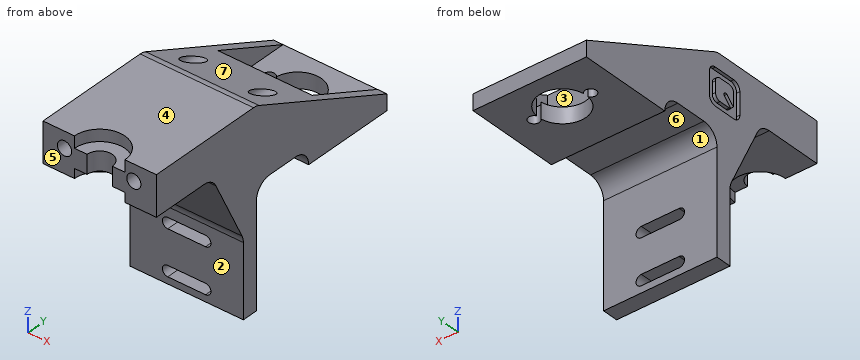
```python
from build123d import *

# Parameters (mm, degrees)
F0_W      = 30
F0_H      = 22
F1_DEPTH  = 5
F2_DEPTH  = 39.1
F3_W      = 30
F3_H      = 12.7
F4_DEPTH  = 50
F8_W      = 30
F8_H      = 5
F9_DEPTH  = 25
F10_W     = 30
F10_H     = 5
F11_DEPTH = 5
F12_W     = 30
F12_H     = 5
F13_DEPTH = 25
F15_DEPTH = 25
F16_DEPTH = 3
F18_DEPTH = 3
F19_DEPTH = 3
F21_DEPTH = 3
F23_DEPTH = 30
F24_R     = 2.25
F25_DEPTH = 500
F26_W     = 68.0921077728
F26_H     = 72.8289508261
F27_DEPTH = 25
F29_DEPTH = 36
F30_R     = 4.99999
F32_DEPTH = 1


# Not quite as in the source:
# - a fillet or chamfer is up to 0.001 mm smaller than in the source, because OpenCascade refuses the exact size


with BuildPart() as f1:
    # F0 (on Front) → F1 (new body)
    with BuildSketch(Plane.XZ):
        with Locations((0, 7.15)):
            Rectangle(F0_W, F0_H)
        with BuildLine():
            ThreePointArc((-6, -1.7), (-7.7, 0), (-6, 1.7))
            Line((-6, 1.7), (6, 1.7))
            ThreePointArc((6, 1.7), (7.7, 0), (6, -1.7))
            Line((6, -1.7), (-6, -1.7))
        make_face(mode=Mode.SUBTRACT)
        with BuildLine():
            ThreePointArc((-6, 12.6), (-7.7, 14.3), (-6, 16))
            Line((-6, 16), (6, 16))
            ThreePointArc((6, 16), (7.7, 14.3), (6, 12.6))
            Line((6, 12.6), (-6, 12.6))
        make_face(mode=Mode.SUBTRACT)
    extrude(amount=F1_DEPTH)

    # F2 (add): a face of the model
    f2_faces = [f1.faces().sort_by_distance(p)[0] for p in [
        (0, -2.5, 18.15),
    ]]
    extrude(f2_faces, amount=F2_DEPTH)

    # F3 (on face) → F4 (join)
    with BuildSketch(Plane.XZ.offset(5)):
        with Locations((0, 50.9)):
            Rectangle(F3_W, F3_H)
    extrude(amount=F4_DEPTH)

    # F6 (on offset) → F7 (revolve, cut)
    with BuildSketch(Plane.XZ.offset(38.3)):
        Polygon((8, 57.25), (0, 57.25), (0, 44.55), (8, 44.55), (8, 47.55), (4, 47.55), (4, 53.55), (8, 53.55), align=None)
    revolve(axis=Axis((0, -38.3, 50.9), (0, 0, 1)), mode=Mode.SUBTRACT)

    # F8 (on face) → F9 (join)
    with BuildSketch(Plane(origin=(0, 0, 0), x_dir=(-1, 0, 0), z_dir=(0, 1, 0))):
        with Locations((0, 36.45)):
            Rectangle(F8_W, F8_H)
    extrude(amount=F9_DEPTH)

    # F10 (on face) → F11 (join)
    with BuildSketch(Plane(origin=(0, 0, 33.95), x_dir=(1, 0, 0), z_dir=(0, 0, -1))):
        with Locations((0, -22.5)):
            Rectangle(F10_W, F10_H)
    extrude(amount=F11_DEPTH)

    # F12 (on face) → F13 (join)
    with BuildSketch(Plane(origin=(0, 25, 0), x_dir=(-1, 0, 0), z_dir=(0, 1, 0))):
        with Locations((0, 31.45)):
            Rectangle(F12_W, F12_H)
    extrude(amount=F13_DEPTH)

    # F14 (on face) → F15 (cut)
    with BuildSketch(Plane.XY.offset(33.95)):
        with BuildLine():
            ThreePointArc((7.4548611111, 38.3216117173), (0, 45), (-7.4548611111, 38.3216117173))
            ThreePointArc((-7.4548611111, 38.3216117173), (-10.75, 37.5), (-7.4548611111, 36.6783882827))
            ThreePointArc((-7.4548611111, 36.6783882827), (0, 30), (7.4548611111, 36.6783882827))
            ThreePointArc((7.4548611111, 36.6783882827), (10.75, 37.5), (7.4548611111, 38.3216117173))
        make_face()
    extrude(amount=-F15_DEPTH, mode=Mode.SUBTRACT)

    # F16 (add): a face of the model
    f16_faces = [f1.faces().sort_by_distance(p)[0] for p in [
        (15, -2.5, -2.6351662665),
    ]]
    extrude(f16_faces, amount=F16_DEPTH)

    # F17 (on face) → F18 (join)
    with BuildSketch(Plane.YZ.offset(18)):
        Polygon((50, 33.95), (0, 57.25), (0, 38.95), (25, 38.95), (25, 33.95), align=None)
    extrude(amount=-F18_DEPTH)

    # F19 (add): a face of the model
    f19_faces = [f1.faces().sort_by_distance(p)[0] for p in [
        (-15, -2.5, -2.6351662665),
    ]]
    extrude(f19_faces, amount=F19_DEPTH)

    # F20 (on face) → F21 (join)
    with BuildSketch(Plane(origin=(-18, 0, 0), x_dir=(0, -1, 0), z_dir=(-1, 0, 0))):
        Polygon((0, 57.25), (-50, 33.95), (-25, 33.95), (-25, 38.95), (0, 38.95), align=None)
    extrude(amount=-F21_DEPTH)

    # F22 (on face) → F23 (join, through all)
    with BuildSketch(Plane(origin=(15, 0, 0), x_dir=(0, -1, 0), z_dir=(-1, 0, 0))):
        Polygon((-25, 45.6), (-25, 38.95), (0, 38.95), (0, 57.25), align=None)
    extrude(amount=F23_DEPTH)

    # F24 (on face) → F25 (cut)
    with BuildSketch(Plane.XZ.offset(55)):
        with Locations((-11.1628601777, 52.1221570671)):
            Circle(F24_R)
        with Locations((10.8371398223, 52.1221570671)):
            Circle(F24_R)
    extrude(amount=-F25_DEPTH, mode=Mode.SUBTRACT)

    # F26 (on offset) → F27 (cut)
    with BuildSketch(Plane.XZ.offset(38.3)):
        with Locations((0.2960525453, 29.3092119973)):
            Rectangle(F26_W, F26_H)
    extrude(amount=F27_DEPTH, mode=Mode.SUBTRACT)

    # F28 (on face) → F29 (join)
    with BuildSketch(Plane(origin=(-18, 0, 0), x_dir=(0, -1, 0), z_dir=(-1, 0, 0))):
        Polygon((5, 44.55), (5, 20.35), (16.9268529862, 44.55), align=None)
    extrude(amount=-F29_DEPTH)

    # F30 (radius 5 in the source; OpenCascade refuses exactly that, so slightly less here)
    f30_edges = [f1.edges().sort_by_distance(p)[0] for p in [
        (0, -16.926853, 44.55),
        (0, 0, 57.25),
        (0, 20, 33.95),
        (0, 0, 33.95),
        (0, -5, 20.35),
    ]]
    fillet(f30_edges, radius=F30_R)

    # F31 (on face) → F32 (cut)
    with BuildSketch(Plane(origin=(-18, 0, 0), x_dir=(0, -1, 0), z_dir=(-1, 0, 0))):
        with BuildLine():
            ThreePointArc((-2.9166666459, 43.103029569), (-2.2332491353, 41.4531137462), (-0.5833333125, 40.7696962357))
            Line((-0.5833333125, 40.7696962357), (6.4166666875, 40.7696962357))
            ThreePointArc((6.4166666875, 40.7696962357), (8.0665825102, 41.4531137462), (8.7500000208, 43.103029569))
            Line((8.7500000208, 43.103029569), (8.7500000208, 50.103029569))
            ThreePointArc((8.7500000208, 50.103029569), (8.0665825102, 51.7529453918), (6.4166666875, 52.4363629023))
            Line((6.4166666875, 52.4363629023), (-0.5833333125, 52.4363629023))
            ThreePointArc((-0.5833333125, 52.4363629023), (-2.2332491353, 51.7529453918), (-2.9166666459, 50.103029569))
            Line((-2.9166666459, 50.103029569), (-2.9166666459, 43.103029569))
        make_face()
        with BuildLine():
            Line((4.6666666875, 43.103029569), (1.1666666875, 43.103029569))
            ThreePointArc((1.1666666875, 43.103029569), (-0.0707701796, 43.6155927019), (-0.5833333125, 44.853029569))
            Line((-0.5833333125, 44.853029569), (-0.5833333125, 48.353029569))
            ThreePointArc((-0.5833333125, 48.353029569), (-0.0707701796, 49.5904664361), (1.1666666875, 50.103029569))
            Line((1.1666666875, 50.103029569), (4.6666666875, 50.103029569))
            ThreePointArc((4.6666666875, 50.103029569), (5.9041035545, 49.5904664361), (6.4166666875, 48.353029569))
            Line((6.4166666875, 48.353029569), (6.4166666875, 44.853029569))
            ThreePointArc((6.4166666875, 44.853029569), (6.3861771815, 44.5277855668), (6.2957710749, 44.2138747406))
            Line((6.2957710875, 44.2138747357), (3.8241204375, 46.6855253857))
            ThreePointArc((3.8241204265, 46.6855253747), (3.4116414708, 46.8563797523), (2.9991625151, 46.6855253747))
            Line((2.9991625041, 46.6855253857), (2.9166666875, 46.603029569))
            Line((2.9166666875, 46.603029569), (2.8341708708, 46.5205337523))
            ThreePointArc((2.8341708818, 46.5205337413), (2.6633165041, 46.1080547857), (2.8341708818, 45.69557583))
            Line((2.8341708708, 45.695575819), (5.3058215208, 43.223925169))
            ThreePointArc((5.3058215159, 43.2239251815), (4.9919106896, 43.133519075), (4.6666666875, 43.103029569))
        make_face(mode=Mode.SUBTRACT)
    extrude(amount=-F32_DEPTH, mode=Mode.SUBTRACT)


solid = f1.part
```
Build history of the part. All positions in model axes, mm. Face numbers are marked on the shaded views. A direction names the side the tool comes from. Give positions to 0.01 mm unless a question says otherwise; leave off trailing zeros. Loops run counter-clockwise (first coordinate to the right, second up) from the corner with the lowest first, then second, coordinate; pieces in that order, holes last. Notation, with made-up numbers: (0, 74.25) -> (30, 74.25) arc R26 cw to (30, 103.25) -> close; hole circle Ø10 at (42.25, 55.5). An arc over 180 degrees is marked (long way). One line per question, with ' | ' between items. Start each with the question number.
1) Cut at C-C (y = -14.5). Give the cut face in (x, z).
2) Cut at D-D (z = 39). Give the cut face in (x, y).
3) Two-plate mould, pull along Y, no slides. Class the marked faces 4, 5, 6 and 7: released by +Y, released by -Y, zero draft, split by the parting line, or undercut.
4) Cut at B-B (x = 0). Count the separate pieces of the cut face and the enclosed holes in it, plus the area to 3 significant figures.
5) Cut at A-A (z = 14.3). Give the cut face in (x, y), plus the area to 3 significant figures.
6) Pin check, flat tips, straight feed: pin 1 (5 mm diameter, centred on x = 0.5, y = 11.5, fed in from -Z); pin 2 (5 mm diameter, centred on x = -7, y = -28.5, fed in from -Z); pin 3 (15 mm diameter, centred on x = -1, y = 36, fed in from -Z); pin 4 (4 mm diameter, centred on x = 10.84, z = 52.12, fed in from +Y). Stop position of each tip, or through.
7) 3-axis set-ups, long thin cutter, end or side, ignore diameter. For the marked faces 1, 2 and 3: which of +Z, -Z, +X, -X, +Y, -Y reach the whole face in a straight line?
8) Probe L1, parallel to X at y = 37.5, z = 31.15; L2, parallel to Y at x = -9, z = 31; L3, parallel to Y at x = -8, z = 15. List the from-to ranges inside material, lowest first.
Return value:
1) outline: (-18, 39.63) -> (18, 39.63) -> (18, 57.25) -> (-18, 57.25) -> close; hole circle Ø4.5 at (-11.16, 52.12); hole circle Ø4.5 at (10.84, 52.12)
2) outline: (-18, -14.19) -> (18, -14.19) -> (18, 39.16) -> (15, 39.16) -> (15, 25) -> (-15, 25) -> (-15, 39.16) -> (-18, 39.16) -> close
3) face 4: zero draft | face 5: released by -Y | face 6: undercut | face 7: released by +Y
4) separate pieces: 4 | enclosed holes: 0 | area: 1,290 mm^2
5) outline: (-18, -5) -> (-7.7, -5) -> (-7.7, 0) -> (-18, 0) -> close; (7.7, -5) -> (18, -5) -> (18, 0) -> (7.7, 0) -> close | area: 103 mm^2
6) pin 1: z = 33.95 | pin 2: z = 44.55 | pin 3: z = 28.95 | pin 4: through
7) face 1: -Z, +X, -X | face 2: -Z, +X, -X, -Y | face 3: +Z, +Y
8) L1: -18 to -10.75, 10.75 to 18 | L2: -10.25 to 0.44, 19.56 to 35.75, 39.25 to 50 | L3: -5 to 0
